Design review of the part built by this model. Coordinates are the model's own, in mm. A direction names the side the tool comes from. Round coordinates to 2 decimals unless told otherwise and drop trailing zeros. Write each loop counter-clockwise with the first axis right and the second up, starting at its lowest first coordinate (ties: lowest second). Pieces come first, ordered by that corner, then holes. Notation, with made-up numbers: (-29.75, 5.25) -> (-20.75, 5.25) arc R32 ccw to (-20.75, 35.25) -> close; hole circle Ø3 at (64, 64). An arc over 180 degrees is marked (long way). One line per question, with ' | ' between items. Start each with the question number.
1) Consider section C-C (y = 3.1). Give the boundary of the cut face in (x, z).
2) Insertion check: pin 1 Ø1.5 at (x, y) = (1.5, 4) entering from -Z; pin 2 Ø2 at (y, z) = (0.5, -3) entering from +X; pin 3 Ø3 at (x, z) = (0.5, -1) entering from -Y. Each pin has a flat end and moves straight along its axis. Give the tip position at first contact, or say it passes through.
3) For probe 1 along Z at (x, y) = (0, 4.95); probe 2 along X at (y, z) = (2.55, 0); probe 3 along Z at (x, y) = (0, 0.1), list the stretches that pass through material, from the lowest coordinate up.
4) Mouldability with a two-part tool opening along X and no side actions: class faces 4 (the cylindrical face through (-1.73, 2.47, 7.81)), 5 (the flat face through (0, 5, 3)), 6 (the cylindrical face through (-0.54, 2.47, 2.44)) as +X half, -X half, draft (parallel to the pull), parting line (faces both ways), or undercut.
5) For faces 1 (the flat face through (1.4, 0.2, -4.2)), 2 (the flat face through (-3, 0, -6)), 3 (the flat face through (1.4, 4.8, 4.2)), list the 3-axis set-ups (+Z, -Z, +X, -X, +Y, -Y) from which the entire face can be reached by the end or side of a thin tool; tool diameter is ignored.
```python
from build123d import *

# Parameters (mm, degrees)
SKETCH1_R           = 8
SKETCH1_R_2         = 2.5
BOSS_EXTRUDE1_DEPTH = 5
SKETCH2_R           = 6.5
SKETCH2_R_2         = 4.2
CUT_EXTRUDE1_DEPTH  = 0.2
SKETCH3_R           = 6.5
SKETCH3_R_2         = 4.2
CUT_EXTRUDE2_DEPTH  = 0.2
CHAMFER1_SIZE       = 0.2


with BuildPart() as part:
    # Sketch1 → Boss-Extrude1 (new body)
    with BuildSketch(Plane(origin=(0, 0, 0), x_dir=(1, 0, 0), z_dir=(0, 1, 0))):
        Circle(SKETCH1_R)
        Circle(SKETCH1_R_2, mode=Mode.SUBTRACT)
    extrude(amount=BOSS_EXTRUDE1_DEPTH)

    # Sketch2 → Cut-Extrude1 (cut)
    with BuildSketch(Plane(origin=(0, 5, 0), x_dir=(1, 0, 0), z_dir=(0, 1, 0))):
        Circle(SKETCH2_R)
        Circle(SKETCH2_R_2, mode=Mode.SUBTRACT)
    extrude(amount=-CUT_EXTRUDE1_DEPTH, mode=Mode.SUBTRACT)

    # Sketch3 → Cut-Extrude2 (cut)
    with BuildSketch(Plane.XZ):
        Circle(SKETCH3_R)
        Circle(SKETCH3_R_2, mode=Mode.SUBTRACT)
    extrude(amount=-CUT_EXTRUDE2_DEPTH, mode=Mode.SUBTRACT)

    # Chamfer1
    chamfer1_edges = [part.edges().sort_by_distance(p)[0] for p in [
        (-8, 0, 0),
        (-8, 5, 0),
        (-2.5, 0, 0),
        (-2.5, 5, 0),
    ]]
    chamfer(chamfer1_edges, length=CHAMFER1_SIZE)


solid = part.part
```
From the geometry:
1) outline: circle Ø16 at (0, 0); hole circle Ø5 at (0, 0)
2) pin 1: stops at z = -7.96 | pin 2: stops at x = 7.75 | pin 3: stops at y = 0.08
3) probe 1: z = -7.85 to -6.5, -4.2 to -2.65, 2.65 to 4.2, 6.5 to 7.85 | probe 2: x = -8 to -2.5, 2.5 to 8 | probe 3: z = -7.9 to -6.5, -4.2 to -2.6, 2.6 to 4.2, 6.5 to 7.9
4) face 4: parting line | face 5: draft | face 6: undercut
5) face 1: -Y | face 2: +Z, -Z, +X, -X, -Y | face 3: +Y
